For this review, take the finished solid that the model builds, in its own axes (mm). A direction names the side the tool comes from. Coordinates: 2 decimals unless noted, no trailing zeros. Loops run counter-clockwise (first coordinate to the right, second up) from the corner with the lowest first, then second, coordinate; pieces in that order, holes last. Notation, with made-up numbers: (17, 83.25) - (72, 83.25) arc R16 cw to (72, 99.25) - close; hole circle Ø10 at (64.25, 17). An arc over 180 degrees is marked (long way). One line per item, written item: value. Start each with the question number.
1. To check wall thickness, follow line 1 (X direction, y = -1.5, z = 0.45); line 2 (X direction, y = -1.5, z = -0.2); line 3 (X direction, y = -1, z = 1.2). State the ranges of each line that lie inside material, in increasing order. Write a range as from..to.
2. Take a section at D-D, the plane x = 2.5. State the section outline as (y, z) points, and give its area (3 significant figures).
3. Take a section at B-B, the plane y = -6. State the section outline as (x, z) points.
4. The part is to be moulded in two halves that separate along X. For faces 1 (the face through (-6, -6.35, 0)), 2 (the face through (5.472, -3.892, 0.219)), say which applies: released by +X, released by -X, zero draft, split by the parting line, or undercut.
5. For faces 3 (the face through (-5.472, -3.822, 0.219)), 4 (the face through (6, -6.35, 0)), list the 3-axis set-ups (+Z, -Z, +X, -X, +Y, -Y) from which the entire face can be reached by the end or side of a thin tool; tool diameter is ignored.
6. Take a section at A-A, the plane z = 0. State the section outline as (x, y) points.
7. Take a section at C-C, the plane y = -2. State the section outline as (x, z) points.
```python
from build123d import *

# Parameters (mm, degrees)
SKETCH1_R           = 2.6035
BOSS_EXTRUDE1_DEPTH = 4.6355
SKETCH3_R           = 0.5715


with BuildPart() as part:
    # Sketch1 → Boss-Extrude1 (new, symmetric)
    with BuildSketch(Plane(origin=(0, 0, 0), x_dir=(0, 0, -1), z_dir=(1, 0, 0))):
        Circle(SKETCH1_R)
    extrude(amount=BOSS_EXTRUDE1_DEPTH, both=True)

    # Sweep1: sweep along a path in Sketch2
    with BuildLine(Plane.XY) as sweep1_path:
        Line((-6, -6.35), (-6, -1.3645))
        ThreePointArc((-6, -1.3645), (-5.600347203, -0.399652797), (-4.6355, 0))
        Line((-4.6355, 0), (4.6355, 0))
        ThreePointArc((4.6355, 0), (5.600347203, -0.399652797), (6, -1.3645))
        Line((6, -1.3645), (6, -6.35))
    # Sketch3 → Sweep1 (sweep)
    with BuildSketch(Plane(origin=(-6, -6.35, 0), x_dir=(1, 0, 0), z_dir=(0, 1, 0))):
        Circle(SKETCH3_R)
    sweep(path=sweep1_path.line)


solid = part.part
```
Solutions:
1. line 1: -6.35..-5.65, -4.64..4.64, 5.65..6.35
1. line 2: -6.54..-5.46, -4.64..4.64, 5.46..6.54
1. line 3: -4.64..4.64
2. outline: circle Ø5.21 at (0, 0)
2. area: 21.3 mm2
3. outline: circle Ø1.14 at (-6, 0); circle Ø1.14 at (6, 0)
4. face 1: zero draft
4. face 2: undercut
5. face 3: -Y
5. face 4: +Z, -Z, +X, -X, -Y
6. outline: (-6.57, -6.35) - (-5.43, -6.35) - (-5.43, -1.36) arc R0.79 cw to (-4.64, -0.57) - (-4.64, -2.6) - (4.64, -2.6) - (4.64, -0.57) arc R0.79 cw to (5.43, -1.36) - (5.43, -6.35) - (6.57, -6.35) - (6.57, -1.36) arc R1.94 ccw to (4.64, 0.57) - (4.64, 2.6) - (-4.64, 2.6) - (-4.64, 0.57) arc R1.94 ccw to (-6.57, -1.36) - close
7. outline: circle Ø1.14 at (-6, 0); (-4.64, -1.67) - (4.64, -1.67) - (4.64, 1.67) - (-4.64, 1.67) - close; circle Ø1.14 at (6, 0)
